from build123d import *

# Parameters (mm, degrees)
EXTRUDE_3_DEPTH    = 10
SHELL_START        = -30
SHELL_1_OUTLINE_W  = 27
SHELL_1_OUTLINE_H  = 12
SHELL_1_DEPTH      = 26
HOLE_WIZARD_M4_2_D = 3.3
HOLE_WIZARD_M4_3_D = 3.3
FILLET_2_R         = 1
FILLET_3_R         = 1


# Read off the part's stored shape, not the designer's step: 薄殼1
with BuildPart() as part:
    # 草圖8 → 填料-伸長3 (new, symmetric)
    with BuildSketch(Plane.XY):
        Polygon((-4, 30), (-30, 4), (-30, 0), (0, 0), (0, 30), align=None)
    extrude(amount=EXTRUDE_3_DEPTH, both=True)

    # 薄殼1 outline → 薄殼1 (cut)
    with BuildSketch(Plane.YZ.offset(SHELL_START)):
        with Locations((17.5, 0)):
            Rectangle(SHELL_1_OUTLINE_W, SHELL_1_OUTLINE_H)
    extrude(amount=SHELL_1_DEPTH, mode=Mode.SUBTRACT)

    # M4 螺紋孔2 (through all)
    with Locations(Plane(origin=(0, 4, 0), x_dir=(-1, 0, 0), z_dir=(0, 1, 0))):
        with Locations((17, 0)):
            Hole(HOLE_WIZARD_M4_2_D / 2)

    # M4 螺紋孔3 (through all)
    with Locations(Plane(origin=(-4, 0, 0), x_dir=(0, -1, 0), z_dir=(-1, 0, 0))):
        with Locations((-17, 0)):
            Hole(HOLE_WIZARD_M4_3_D / 2)

    # 圓角2
    fillet_2_edges = [part.edges().sort_by_distance(p)[0] for p in [
        (-4, 17, -6),
        (-4, 17, 6),
        (0, 0, 0),
    ]]
    fillet(fillet_2_edges, radius=FILLET_2_R)

    # 圓角3
    fillet_3_edges = [part.edges().sort_by_distance(p)[0] for p in [
        (-15.5, 0, 10),
        (-17.5, 4, -6),
        (-17.5, 4, 6),
        (-4, 4, 0),
        (-4.292893219, 4, -5.707106781),
        (-4.292893219, 4, 5.707106781),
        (0, 15.5, -10),
        (0, 15.5, 10),
        (-0.292893219, 0.292893219, -10),
        (-0.292893219, 0.292893219, 10),
        (-15.5, 0, -10),
    ]]
    fillet(fillet_3_edges, radius=FILLET_3_R)


solid = part.part
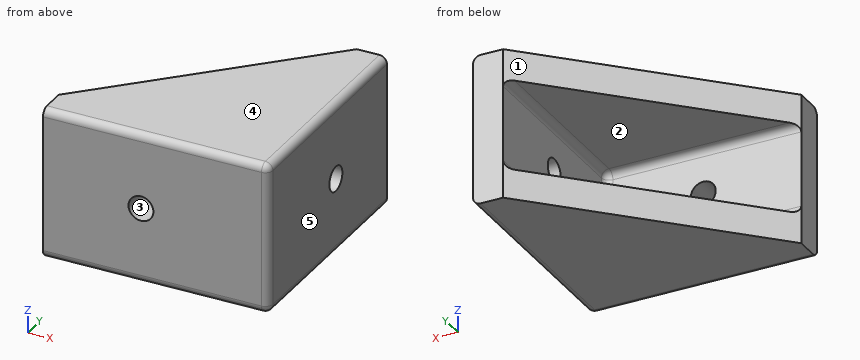
Geometry: final body of the model. Coordinates: model frame, mm. Face numbers are marked on the shaded views. A direction names the side the tool comes from. Give positions to 0.01 mm unless a question says otherwise; leave off trailing zeros. Write each loop counter-clockwise with the first axis right and the second up, starting at its lowest first coordinate (ties: lowest second). Pieces come first, ordered by that corner, then holes.
(1) Cut plane C-C, the plane z = 1.25. Return loops of the section in (x, y).
(2) Cut plane B-B, the plane x = -17. Return loops of the section in (y, z), then the cut area to 3 significant figures.
(3) Access query for the marked faces 1 and 2. Directions: +Z, -Z, +X, -X, +Y, -Y. A direction counts if a zero-diameter tool reaches every point of the face in a straight line with its end or side. Return the directions, or none.
(4) Cut plane D-D, the plane y = 5.5. Return loops of the section in (x, z), then the cut area to 3 significant figures.
(5) Cut plane A-A, the plane y = 17. Return loops of the section in (x, z), then the cut area to 3 significant figures.
(6) Mould query, pull axis X, two halves, no side actions, for the marked faces 3, 4 and 5. Classes: released by +X, released by -X, zero draft, split by the parting line, or undercut.
(7) First-contact query: P1, Ø3, axis at x = -12, z = 1.5, coming from the +Y side; P2, Ø11, axis at y = 16.5, z = 0, coming from the -X side. Flat tips, straight axial feed; report the tip coordinate or a pass-through.
(8) Ray query, line 1 (Z direction, x = -19, y = 5.5); line 2 (Z direction, x = -2.6, y = 17); line 3 (X direction, y = 7.25, z = 3.5). Return the intervals inside material, ascending.
Values follow:
1. outline: (-30, 0) - (-18.08, 0) - (-18.08, 4) - (-30, 4) - close; (-15.92, 0) - (-1, 0) arc R1 ccw to (0, 1) - (0, 15.92) - (-4, 15.92) - (-4, 5) arc R1 cw to (-5, 4) - (-15.92, 4) - close; (-4, 18.08) - (0, 18.08) - (0, 30) - (-4, 30) - close
2. outline: (0, -9) arc R1 ccw to (1, -10) - (17, -10) - (17, -6) - (5, -6) arc R1 cw to (4, -5) - (4, -1.65) - (0, -1.65) - close; (0, 1.65) - (4, 1.65) - (4, 5) arc R1 cw to (5, 6) - (17, 6) - (17, 10) - (1, 10) arc R1 ccw to (0, 9) - close
2. area: 171 mm2
3. face 1: +Z, -Z, -X, +Y
3. face 2: -X, +Y
4. outline: (-28.5, -10) - (-1, -10) arc R1 ccw to (0, -9) - (0, 9) arc R1 ccw to (-1, 10) - (-28.5, 10) - (-28.5, 6) - (-5, 6) arc R1 cw to (-4, 5) - (-4, -5) arc R1 cw to (-5, -6) - (-28.5, -6) - close
4. area: 276 mm2
5. outline: (-17, -10) - (-1, -10) arc R1 ccw to (0, -9) - (0, -1.65) - (-4, -1.65) - (-4, -5) arc R1 cw to (-5, -6) - (-17, -6) - close; (-17, 6) - (-5, 6) arc R1 cw to (-4, 5) - (-4, 1.65) - (0, 1.65) - (0, 9) arc R1 ccw to (-1, 10) - (-17, 10) - close
5. area: 171 mm2
6. face 3: undercut
6. face 4: zero draft
6. face 5: released by +X
7. P1: stops at y = 4
7. P2: stops at x = -4.13
8. line 1: z = -10 to -6, 6 to 10
8. line 2: z = -10 to -1.65, 1.65 to 10
8. line 3: x = -4 to 0
